Here's the drawing with two shaded views (mm, measured from the low corner). I have some questions. A direction names the side the tool comes from. Round coordinates to 2 decimals unless told otherwise and drop trailing zeros. Write each loop counter-clockwise with the first axis right and the second up, starting at its lowest first coordinate (ties: lowest second). Pieces come first, ordered by that corner, then holes. Notation, with made-up numbers: M -40,-19.75 L 3,-19.75 A26 ccw 3,-0.75 Z; hole C -23.5,-10.75 d9. An arc over 180 degrees is marked long. Answer as a JSON object with one key per item and string values. Group by question number.
1) Suppose I cut it at D-D, the plane y = 10. Write out the boundary of the cut face in (x, z).
2) Please list where these lines run through material, in increasing order: L1, parallel to Z at x = 10, y = 1.55; L2, parallel to X at y = 10.25, z = 10.25; L3, parallel to Y at x = 8, z = 8. Write a range as [from, to].
3) Suppose I cut it at A-A, the plane y = 3. Write out the boundary of the cut face in (x, z), and give its area (3 significant figures).
4) On a 3-axis mill with a long thin cutter (end or side, diameter ignored), from which of +Z, -Z, +X, -X, +Y, -Y can I reach the whole of each face in a straight line? I mean the marked faces 4 and 5. Say none if no direction works.
5) Suppose I cut it at B-B, the plane x = 10. Write out the boundary of the cut face in (y, z), and give its area (3 significant figures).
6) I'm going to push flat-ended pins straight in: pin 1 Ø1.5 at (y, z) = (3.5, 5) entering from -X; pin 2 Ø1.5 at (y, z) = (7.5, 2.5) entering from +X; pin 3 Ø1 at (x, z) = (11.5, 9) entering from -Y. Where does each tip first touch, or does it pass through?
7) Suppose I cut it at C-C, the plane z = 10. Write out the boundary of the cut face in (x, y).
8) If we mould it in two halves opening along X, with no side actions, what happens to the marked faces 1, 2 and 3? For each: +X half, -X half, draft (parallel to the pull), parting line (faces both ways), or undercut.
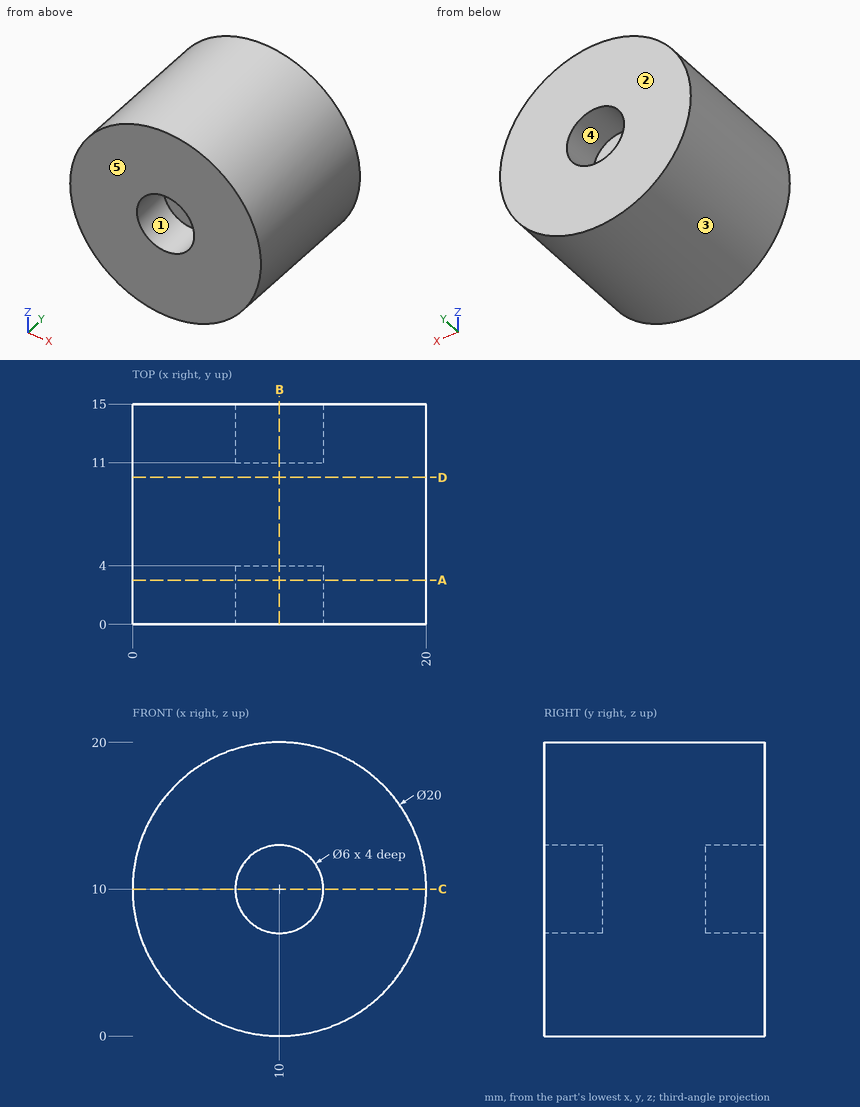
Results:
{
 "1": {"outline": "C 10,10 d20"},
 "2": {"L1": "[0, 7], [13, 20]", "L2": "[0, 20]", "L3": "[4, 11]"},
 "3": {"outline": "C 10,10 d20; hole C 10,10 d6", "area": "286 mm^2"},
 "4": {"face 4": "+Y", "face 5": "+Z, -Z, +X, -X, -Y"},
 "5": {"outline": "M 0,0 L 15,0 L 15,7 L 11,7 L 11,13 L 15,13 L 15,20 L 0,20 L 0,13 L 4,13 L 4,7 L 0,7 Z", "area": "252 mm^2"},
 "6": {"pin 1": "x = 0.95", "pin 2": "x = 17.38", "pin 3": "y = 4"},
 "7": {"outline": "M 0,0 L 7,0 L 7,4 L 13,4 L 13,0 L 20,0 L 20,15 L 13,15 L 13,11 L 7,11 L 7,15 L 0,15 Z"},
 "8": {"face 1": "undercut", "face 2": "draft", "face 3": "parting line"}
}
